Design review of the part built by this model. Coordinates are the model's own, in mm. Face numbers are marked on the shaded views. A direction names the side the tool comes from. Coordinates: 2 decimals unless noted, no trailing zeros. Loops run counter-clockwise (first coordinate to the right, second up) from the corner with the lowest first, then second, coordinate; pieces in that order, holes last. Notation, with made-up numbers: M 8.25,42.25 L 38.25,42.25 A29 cw 38.25,76.25 Z; hole C 58.5,0 d1. An arc over 180 degrees is marked long. Put each result on its own line as item: value. Start each with the question number.
(1) For the marked faces 5 and 6, list the 3-axis set-ups (+Z, -Z, +X, -X, +Y, -Y) from which the entire face can be reached by the end or side of a thin tool; tool diameter is ignored.
(2) Take a section at B-B, the plane y = 221. Give the boundary of the cut face in (x, z).
(3) Take a section at C-C, the plane x = 119. Give the boundary of the cut face in (y, z).
(4) The part is to be moulded in two halves that separate along X. For the marked faces 1, 2, 3 and 4, say which applies: +X half, -X half, draft (parallel to the pull), parting line (faces both ways), or undercut.
(5) For probe 1 along X at (y, z) = (89, -1); probe 2 along Y at (x, z) = (-295, -210), list the stretches that pass through material, from the lowest coordinate up. Write a range as [from, to].
(6) Take a section at D-D, the plane z = 13.5. Give the boundary of the cut face in (x, y).
(7) Take a section at A-A, the plane z = 210. Give the boundary of the cut face in (x, y), then the cut area to 3 significant figures.
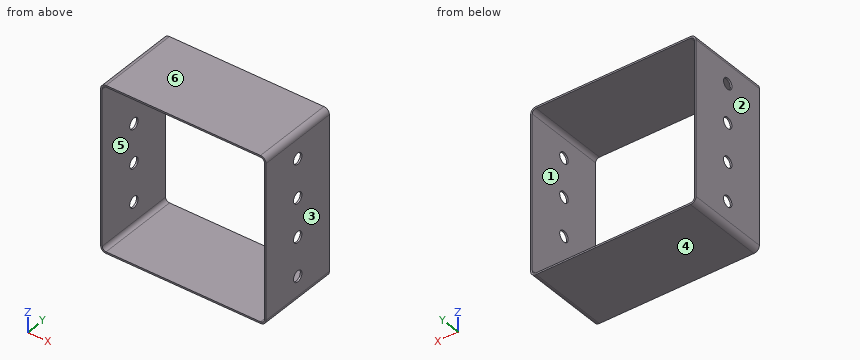
Autodesk Inventor part; units mm, degrees
ref_plane "YZ Plane" through (0, 0, 0) normal (1, 0, 0) x (0, 1, 0)
ref_plane "XZ Plane" through (0, 0, 0) normal (0, 1, 0) x (-1, 0, 0)
ref_plane "XY Plane" through (0, 0, 0) normal (0, 0, 1) x (1, 0, 0)
sketch "Sketch1" plane through (0, 0, 0) normal (0, 1, 0) x (-1, 0, 0)
  line L0 (-280, 300) -> (280, 300)
  line L1 (300, 280) -> (300, -280)
  line L2 (280, -300) -> (-280, -300)
  line L3 (-300, -280) -> (-300, 280)
  line L4 (-300, 300) -> (300, -300) construction
  line L5 (300, 300) -> (-300, -300) construction
  arc A0 (300, 280) -> (280, 300) centre (280, 280) ccw
  arc A1 (280, -300) -> (300, -280) centre (280, -280) ccw
  arc A2 (-300, -280) -> (-280, -300) centre (-280, -280) ccw
  arc A3 (-280, 300) -> (-300, 280) centre (-280, 280) ccw
  line L6 (280, 294) -> (-280, 294)
  arc A4 (-280, 294) -> (-294, 280) centre (-280, 280) ccw
  line L7 (-294, 280) -> (-294, -280)
  arc A5 (-294, -280) -> (-280, -294) centre (-280, -280) ccw
  line L8 (-280, -294) -> (280, -294)
  arc A6 (280, -294) -> (294, -280) centre (280, -280) ccw
  line L9 (294, -280) -> (294, 280)
  arc A7 (294, 280) -> (280, 294) centre (280, 280) ccw
  point P0 (0, 0)
  dimension "d0" = 600
  dimension "d1" = 600
  dimension "d2" = 20
  dimension "d3" = 6
extrude "Extrusion1" add sketch "Sketch1" along normal blind 300
sketch "Sketch2" plane through (300, 0, 280) normal (1, 0, 0) x (0, 0, -1)
  line L0 (0, 0) -> (0, 300)
  line L1 (0, 150) -> (560, 150) construction
  line L2 (560, 0) -> (560, 300)
  point P0 (280, 0)
  point P1 (70, 150)
  point P2 (210, 150)
  point P3 (350, 150)
  point P4 (490, 150)
  dimension "d6" = 70
  dimension "d7" = 140
  dimension "d8" = 140
  dimension "d9" = 140
hole "Hole1" at (300, 150, 210) at (300, 150, 70) at (300, 150, -70) at (300, 150, -210) direction (-1, 0, 0) diameter 40 end through all
properties part number "Stackbox"
Computed values:
1. face 5: +Y, -Y
1. face 6: +Z, +X, -X, +Y, -Y
2. outline: M -300,-280 A20 ccw -280,-300 L 280,-300 A20 ccw 300,-280 L 300,280 A20 ccw 280,300 L -280,300 A20 ccw -300,280 Z; hole M -294,-280 A14 ccw -280,-294 L 280,-294 A14 ccw 294,-280 L 294,280 A14 ccw 280,294 L -280,294 A14 ccw -294,280 Z
3. outline: M 0,-300 L 300,-300 L 300,-294 L 0,-294 Z; M 0,294 L 300,294 L 300,300 L 0,300 Z
4. face 1: undercut
4. face 2: -X half
4. face 3: +X half
4. face 4: draft
5. probe 1: x = [-300, -294], [294, 300]
5. probe 2: y = [0, 130], [170, 300]
6. outline: M -300,0 L -294,0 L -294,300 L -300,300 Z; M 294,0 L 300,0 L 300,300 L 294,300 Z
7. outline: M -300,0 L -294,0 L -294,130 L -300,130 Z; M -300,170 L -294,170 L -294,300 L -300,300 Z; M 294,0 L 300,0 L 300,130 L 294,130 Z; M 294,170 L 300,170 L 300,300 L 294,300 Z
7. area: 3,120 mm^2
